```python
from build123d import *

# Parameters (mm, degrees)
F0_R     = 15
F1_DEPTH = 25


with BuildPart() as f1:
    # F0 (on Front) → F1 (new body)
    with BuildSketch(Plane.XZ):
        with BuildLine():
            Line((474.8, 142.5), (-7.281521, 31.673798))
            ThreePointArc((-7.281521, 31.673798), (-32.292789, -3.664122), (0, -32.5))
            Line((0, -32.5), (474.8, -32.5))
            Line((474.8, -32.5), (474.8, 55))
            Line((474.8, 55), (499.8, 55))
            Line((499.8, 55), (499.8, -32.5))
            Line((499.8, -32.5), (637.3, -32.5))
            Line((637.3, -32.5), (637.3, 117.5))
            Line((637.3, 117.5), (499.8, 117.5))
            Line((499.8, 117.5), (499.8, 142.5))
            Line((499.8, 142.5), (474.8, 142.5))
        make_face()
        with BuildLine():
            ThreePointArc((14.741868, 2.770801), (14.935328, 1.391399), (15, 0))
            ThreePointArc((15, 0), (-14.935328, -1.391399), (14.741868, 2.770801))
        make_face(mode=Mode.SUBTRACT)
        with Locations((67.162807, 10.637544)):
            Circle(F0_R, mode=Mode.SUBTRACT)
        with Locations((134.325614, 21.275087)):
            Circle(F0_R, mode=Mode.SUBTRACT)
        with Locations((201.488421, 31.912631)):
            Circle(F0_R, mode=Mode.SUBTRACT)
        with Locations((268.651229, 42.550174)):
            Circle(F0_R, mode=Mode.SUBTRACT)
        with Locations((335.814036, 53.187718)):
            Circle(F0_R, mode=Mode.SUBTRACT)
        with Locations((402.976843, 63.825262)):
            Circle(F0_R, mode=Mode.SUBTRACT)
    extrude(amount=F1_DEPTH)


solid = f1.part
```
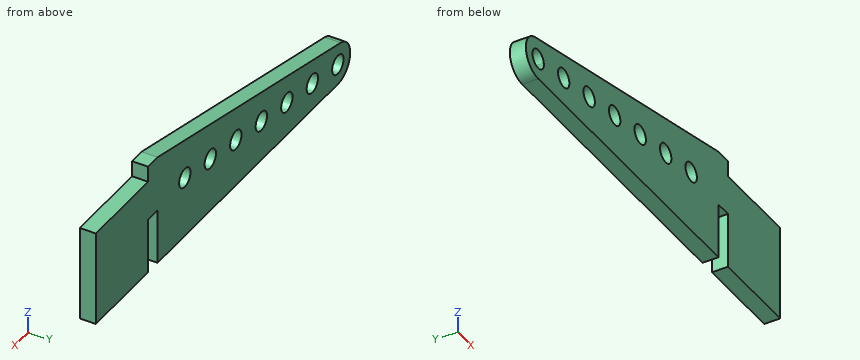
Build history of the part. All positions in model axes, mm. Coordinates: 2 decimals unless noted, no trailing zeros. Write each loop counter-clockwise with the first axis right and the second up, starting at its lowest first coordinate (ties: lowest second). Pieces come first, ordered by that corner, then holes.
1. Drop flat-ended pins along their axis: pin 1 (12.5 mm diameter, centred on y = -15, z = 125, fed in from +X); pin 2 (18 mm diameter, centred on x = 67.16, z = 10.64, fed in from -Y); pin 3 (7.5 mm diameter, centred on x = 485.5, y = -12.5, fed in from -Z); pin 4 (12.5 mm diameter, centred on x = 540, y = -16, fed in from +Z). Give the stop position or say it passes through.
Answer block:
pin 1: stops at x = 499.8
pin 2: passes through
pin 3: stops at z = 55
pin 4: stops at z = 117.5
2. Drill centre lines: probe 1 along X at (y, z) = (-9.5, 16); probe 2 along Z at (x, y) = (415, -5); probe 3 along X at (y, z) = (-21.5, 27). Where is each one in solid material? Low to high.
Answer block:
probe 1: x = -28.29 to 53.15, 81.17 to 120.28, 148.37 to 474.8, 499.8 to 637.3
probe 2: z = -32.5 to 54.86, 72.79 to 128.75
probe 3: x = -18.09 to 120.46, 148.19 to 187.32, 215.66 to 474.8, 499.8 to 637.3
3. Band-saw the part on C-C, the plane z = 97. Give the cut face in (x, y).
Answer block:
outline: (276.88, -25) - (637.3, -25) - (637.3, 0) - (276.88, 0) - close
4. Band-saw the part on B-B, the plane x = 482. Give the cut face in (y, z), and give its area (3 significant figures).
Answer block:
outline: (-25, 55) - (0, 55) - (0, 142.5) - (-25, 142.5) - close
area: 2,190 mm2
5. Band-saw the part on A-A, the plane y = -11. Give the cut face in (x, z), and give its area (3 significant figures).
Answer block:
outline: (-7.28, 31.67) arc R32.5 ccw to (0, -32.5) - (474.8, -32.5) - (474.8, 55) - (499.8, 55) - (499.8, -32.5) - (637.3, -32.5) - (637.3, 117.5) - (499.8, 117.5) - (499.8, 142.5) - (474.8, 142.5) - close; hole (14.74, 2.77) arc R15 ccw (long way) to (15, 0) arc R15 ccw to start; hole circle Ø30 at (67.16, 10.64); hole circle Ø30 at (134.33, 21.28); hole circle Ø30 at (201.49, 31.91); hole circle Ø30 at (268.65, 42.55); hole circle Ø30 at (335.81, 53.19); hole circle Ø30 at (402.98, 63.83)
area: 76,700 mm2
